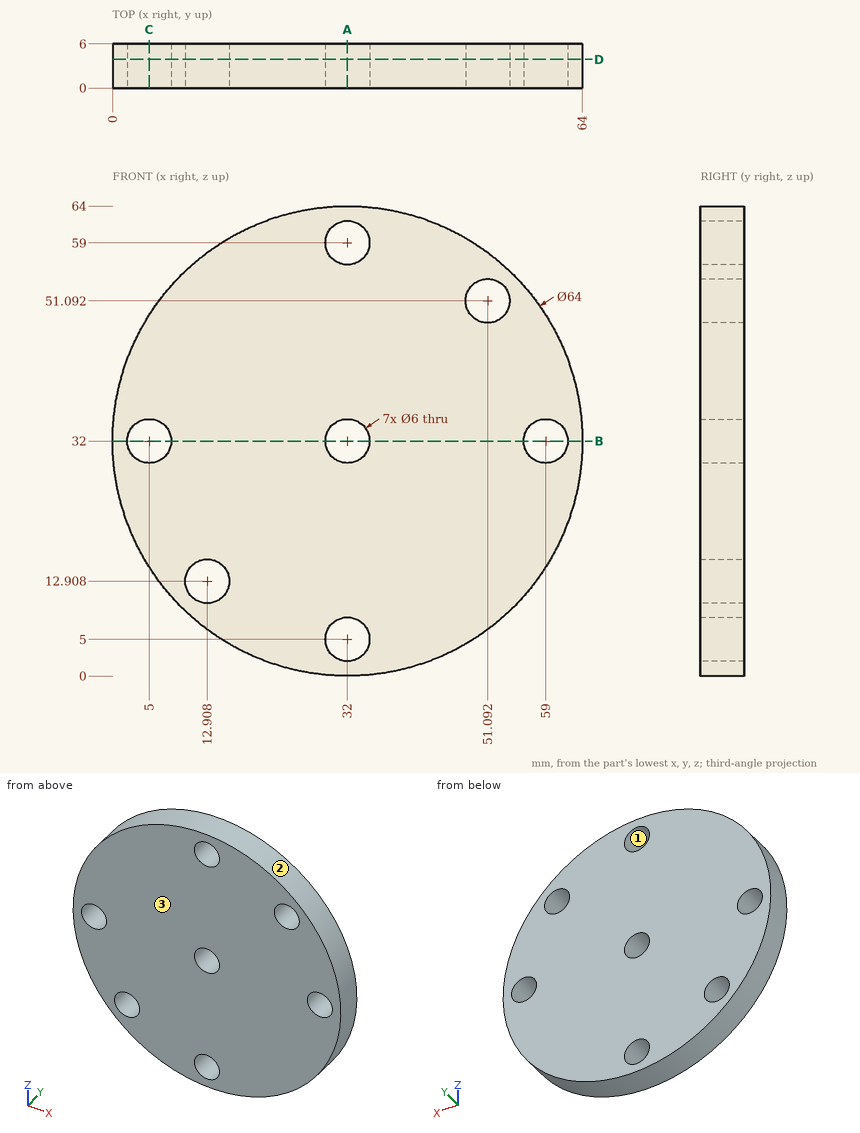
Job drawing, mm, ordinate dimensions from the low corner. One solid piece. Coordinates: 2 decimals unless noted, no trailing zeros. Order: outer loops, then holes, each group sorted by start corner. A loop starts at its lowest first (then second) coordinate and runs counter-clockwise, first axis right, second up. Notation, with made-up numbers: (39, 5.25) - (90, 5.25) arc R16 ccw to (90, 32.25) - close; hole circle Ø8 at (-3, 26.5). An arc over 180 degrees is marked (long way). Return JSON: item names as keys, results as strings. Group by question number.
1) Saw through at C-C, the plane x = 5. Write the cut outline in (y, z), plus the area to 3 significant figures.
2) Saw through at D-D, the plane y = 3.9. Write the cut outline in (x, z), plus the area to 3 significant figures.
3) Flat gauge pins, fed straight in: P1, Ø7, axis at x = 51.09, z = 51.09, coming from the +Y side; P2, Ø2, axis at y = 3.5, z = 20.5, coming from the -X side; P3, Ø1, axis at x = 38, y = 3, coming from the +Z side; P4, Ø3.5, axis at x = 32, z = 5, coming from the +Y side. Where does each tip first touch, or does it go through?
4) Saw through at A-A, the plane x = 32. Write the cut outline in (y, z).
5) Mould opens along X. For the marked faces 1, 2 and 3 say: released by +X, released by -X, zero draft, split by the parting line, or undercut.
6) Saw through at B-B, the plane z = 32. Write the cut outline in (x, y), plus the area to 3 significant figures.
7) Probe line 1 (Z direction, x = 33.5, y = 1.25) (1 decimal); line 2 (Z direction, x = 13, y = 3.35); line 3 (X direction, y = 5.3, z = 52.5). List the from-to ranges inside material, lowest first. Write a range as from..to.
Values found:
{
 "1": {"outline": "(0, 14.82) - (6, 14.82) - (6, 29) - (0, 29) - close; (0, 35) - (6, 35) - (6, 49.18) - (0, 49.18) - close", "area": "170 mm²"},
 "2": {"outline": "circle Ø64 at (32, 32); hole circle Ø6 at (5, 32); hole circle Ø6 at (12.91, 12.91); hole circle Ø6 at (32, 5); hole circle Ø6 at (32, 32); hole circle Ø6 at (32, 59); hole circle Ø6 at (51.09, 51.09); hole circle Ø6 at (59, 32)", "area": "3,020 mm²"},
 "3": {"P1": "stops at y = 6", "P2": "stops at x = 1.77", "P3": "stops at z = 63.52", "P4": "passes through"},
 "4": {"outline": "(0, 0) - (6, 0) - (6, 2) - (0, 2) - close; (0, 8) - (6, 8) - (6, 29) - (0, 29) - close; (0, 35) - (6, 35) - (6, 56) - (0, 56) - close; (0, 62) - (6, 62) - (6, 64) - (0, 64) - close"},
 "5": {"face 1": "undercut", "face 2": "split by the parting line", "face 3": "zero draft"},
 "6": {"outline": "(0, 0) - (2, 0) - (2, 6) - (0, 6) - close; (8, 0) - (29, 0) - (29, 6) - (8, 6) - close; (35, 0) - (56, 0) - (56, 6) - (35, 6) - close; (62, 0) - (64, 0) - (64, 6) - (62, 6) - close", "area": "276 mm²"},
 "7": {"line 1": "z = 0..2.4, 7.6..29.4, 34.6..56.4, 61.6..64", "line 2": "z = 6.25..9.91, 15.91..57.75", "line 3": "x = 7.43..48.44, 53.74..56.57"}
}
